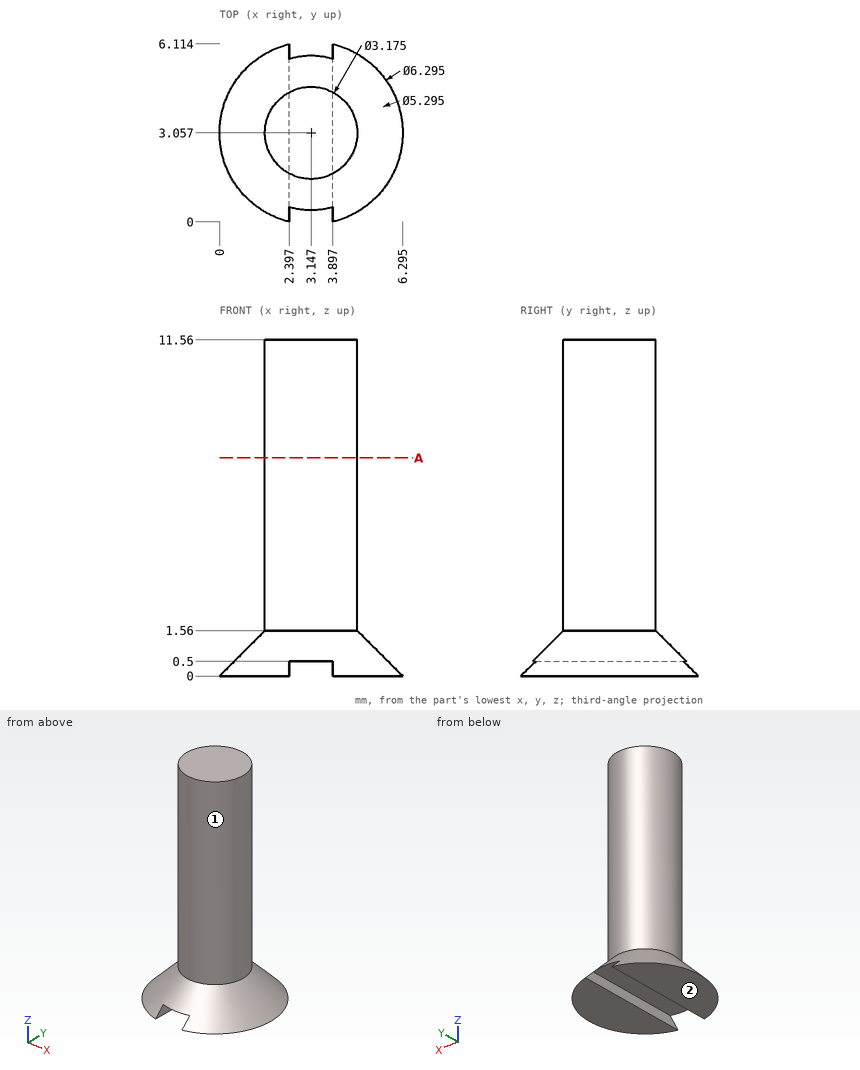
Answer from the drawing. Dimensions are ordinates in mm from the lowest x, y and z of the part. A direction names the side the tool comes from. Round coordinates to 2 decimals unless told otherwise and drop trailing zeros. Write each loop counter-clockwise with the first axis right and the second up, starting at its lowest first coordinate (ties: lowest second). Pieces come first, ordered by that corner, then holes. Notation, with made-up numbers: (-10, -20) - (35, -20) arc R16 cw to (35, -13) - close; hole circle Ø6 at (47.5, 1.5). An arc over 180 degrees is marked (long way). Use a Markdown table: item, result.
(1) Which of the six approach directions +Z, -Z, +X, -X, +Y, -Y give full straight-line access (tool end or side, diameter ignored) to the marked faces 1 and 2?
Reported:
| item | result |
|---|---|
| face 1 | +Z |
| face 2 | -Z, +X, -X, +Y, -Y |
(2) Each of these flat-tipped pins is pushed along its axis until it touches: pin 1 Ø1 at (y, z) = (2, 5.5) entering from -X; pin 2 Ø0.6 at (y, z) = (1.5, 0) entering from +X; pin 3 Ø2 at (x, y) = (3, 1) entering from -Z. Where does it stop, or does it pass through?
Reported:
| item | result |
|---|---|
| pin 1 | x = 1.66 |
| pin 2 | x = 6.03 |
| pin 3 | z = 0 |
(3) Straight lines are drawn through the part: line 1 along X through (y, z) = (3.5, 1.5) (1 decimal); line 2 along Z through (x, y) = (3.75, 4.25); line 3 along Y through (x, z) = (2, 7) (1 decimal). For each, find the intervals that lie inside material, in ascending order. Write a range as [from, to].
Reported:
| item | result |
|---|---|
| line 1 | [1.6, 4.7] |
| line 2 | [0.5, 11.56] |
| line 3 | [2, 4.2] |
(4) The part is cut by section A-A (z = 7.5). Write down the section's boundary in (x, y) (1 decimal).
Reported:
| item | result |
|---|---|
| outline | circle Ø3.2 at (3.1, 3.1) |
